from build123d import *
from OCP.BRepFilletAPI import BRepFilletAPI_MakeChamfer

# Parameters (mm, degrees)
SKETCH1_R           = 24
BOSS_EXTRUDE1_DEPTH = 2
CHAMFER1_SIZE       = 2
CHAMFER1_SIZE_2     = 1.5
SKETCH3_R           = 3
SKETCH3_R_2         = 1.5
CUT_EXTRUDE1_DEPTH  = 2
CHAMFER2_SIZE       = 0.8
CHAMFER2_SIZE_2     = 2
CHAMFER3_SIZE       = 1.86


# Some blends are built 0.0001 mm under size
with BuildPart() as part:
    # Sketch1 → Boss-Extrude1 (new body)
    with BuildSketch(Plane.XY):
        Polygon((38.85, -60), (38.85, 50), (-7.5, 50), (-34.847350762, 40.623765453), (-39.5, 36.014047515), (-39.5, -39.169048105), (-27.001428863, -60), align=None)
        Circle(SKETCH1_R, mode=Mode.SUBTRACT)
    extrude(amount=BOSS_EXTRUDE1_DEPTH)

    # Chamfer1
    chamfer1_edges_1 = [part.edges().sort_by_distance(p)[0] for p in [
        (-39.5, -1.577500295, 2),
    ]]
    chamfer1_side_1 = [part.faces().sort_by_distance(p)[0] for p in [
        (-39.5, -1.577500295, 1.97),
    ]]
    chamfer1_edges_2 = [part.edges().sort_by_distance(p)[0] for p in [
        (-33.250714432, -49.584524053, 2),
    ]]
    chamfer1_side_2 = [part.faces().sort_by_distance(p)[0] for p in [
        (-33.250714432, -49.584524053, 1.97),
    ]]
    chamfer1_edges_3 = [part.edges().sort_by_distance(p)[0] for p in [
        (-37.173675381, 38.318906484, 2),
    ]]
    chamfer1_side_3 = [part.faces().sort_by_distance(p)[0] for p in [
        (-37.173675381, 38.318906484, 1.97),
    ]]
    chamfer1 = BRepFilletAPI_MakeChamfer(part.part.solid().wrapped)
    for e in chamfer1_edges_1:
        chamfer1.Add(CHAMFER1_SIZE - 0.0001, CHAMFER1_SIZE_2 - 0.0001, e.wrapped, chamfer1_side_1[0].wrapped)
    for e in chamfer1_edges_2:
        chamfer1.Add(CHAMFER1_SIZE - 0.0001, CHAMFER1_SIZE_2 - 0.0001, e.wrapped, chamfer1_side_2[0].wrapped)
    for e in chamfer1_edges_3:
        chamfer1.Add(CHAMFER1_SIZE - 0.0001, CHAMFER1_SIZE_2 - 0.0001, e.wrapped, chamfer1_side_3[0].wrapped)
    add(Compound.cast(chamfer1.Shape()), mode=Mode.REPLACE)  # a hair under: the kernel refuses the full size

    # Sketch3 → Cut-Extrude1 (cut)
    with BuildSketch(Plane.XY.offset(2)):
        with Locations((2.5, 40)):
            Circle(SKETCH3_R)
        with Locations((-19.291144984, -54)):
            Circle(SKETCH3_R_2)
        with Locations((25.5, -54)):
            Circle(SKETCH3_R_2)
        with Locations((25.5, 44)):
            Circle(SKETCH3_R_2)
        with Locations((-28.642921649, 36.408141149)):
            Circle(SKETCH3_R_2)
    extrude(amount=-CUT_EXTRUDE1_DEPTH, mode=Mode.SUBTRACT)

    # Chamfer2
    # the kernel refuses this chamfer: 2, 0.8 mm, written as the material it takes off along each edge
    with BuildSketch(Plane(origin=(-30.438487192, -60, 2), x_dir=(0, 0.996016754004022, 0.08916628142572558), z_dir=(1, 0, 0))) as chamfer2_piece_1:
        Polygon((CHAMFER2_SIZE * 0.996016754004, -CHAMFER2_SIZE * 0.0891662814257), (-CHAMFER2_SIZE_2 * 0.0891662814257, -CHAMFER2_SIZE_2 * 0.996016754004), (0, 0), align=None)
    extrude(amount=74.47471447, mode=Mode.SUBTRACT)
    with BuildSketch(Plane(origin=(44.036227278, 50, 2), x_dir=(0, -0.996016754004022, 0.08916628142572558), z_dir=(-1, 0, 0))) as chamfer2_piece_2:
        Polygon((CHAMFER2_SIZE * 0.996016754004, -CHAMFER2_SIZE * 0.0891662814257), (-CHAMFER2_SIZE_2 * 0.0891662814257, -CHAMFER2_SIZE_2 * 0.996016754004), (0, 0), align=None)
    extrude(amount=56.722454557, mode=Mode.SUBTRACT)
    with BuildSketch(Plane(origin=(-2.594109331, 51.682019658, 2), x_dir=(-0.0046450347702198845, 0.013548018079808006, -0.9998974321689664), z_dir=(-0.945945945945946, -0.3243243243243241, 0))) as chamfer2_piece_3:
        Polygon((CHAMFER2_SIZE_2 * 0.999897432169, CHAMFER2_SIZE_2 * 0.0143221905415), (-CHAMFER2_SIZE * 0.0143221905415, CHAMFER2_SIZE * 0.999897432169), (0, 0), align=None)
    extrude(amount=35.83751357, mode=Mode.SUBTRACT)

    # Chamfer3
    chamfer3_edges = [part.edges().sort_by_distance(p)[0] for p in [
        (-20.791144984, -54, 2),
        (24, -54, 2),
        (24, 44, 2),
        (-30.142921649, 36.408141149, 2),
    ]]
    chamfer(chamfer3_edges, length=CHAMFER3_SIZE)


solid = part.part
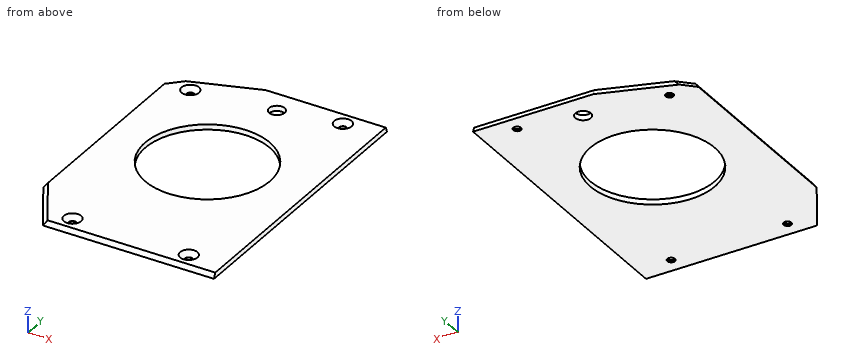
The listing builds one solid part. Answer for the finished solid, in the listing's coordinates (mm). Give positions to 0.01 mm unless a question says otherwise; leave off trailing zeros. Loops run counter-clockwise (first coordinate to the right, second up) from the corner with the lowest first, then second, coordinate; pieces in that order, holes last.
Item 1: A cutting plane is placed at B-B (x = 25.5). Give the vertices of the cut face in (y, z).
Derived:
outline: (-60, 0) - (-55.5, 0) - (-55.5, 0.14) - (-57.36, 2) - (-59.2, 2) - close; (-52.5, 0) - (42.5, 0) - (42.5, 0.14) - (40.64, 2) - (-50.64, 2) - (-52.5, 0.14) - close; (45.5, 0) - (50, 0) - (49.2, 2) - (47.36, 2) - (45.5, 0.14) - close
Item 2: A cutting plane is placed at D-D (y = -54). Give the number of separate pieces and of enclosed holes in the cut face, then the cut area to 3 significant figures.
Derived:
separate pieces: 3
enclosed holes: 0
area: 118 mm2
Item 3: Find the intervals of material crossed by line 1 along Y through (x, z) = (0, 1.2); line 2 along X through (y, z) = (-54, 0.75); line 3 along Y through (x, z) = (2.5, 0.2), in increasing order.
Derived:
line 1: y = -59.52 to -24, 24 to 38.34, 41.66 to 49.52
line 2: x = -29.95 to -21.4, -17.18 to 23.39, 27.61 to 38.85
line 3: y = -59.92 to -23.87, 23.87 to 37, 43 to 49.92
Item 4: A cutting plane is placed at C-C (z = 0.6). Give the vertices of the cut face in (x, y).
Derived:
outline: (-39.05, -39.04) - (-26.62, -59.76) - (38.85, -59.76) - (38.85, 49.76) - (-7.46, 49.76) - (-34.26, 40.57) - (-39.05, 35.83) - close; hole circle Ø3.92 at (-28.64, 36.41); hole circle Ø48 at (0, 0); hole circle Ø3.92 at (-19.29, -54); hole circle Ø6 at (2.5, 40); hole circle Ø3.92 at (25.5, -54); hole circle Ø3.92 at (25.5, 44)
